```python
from build123d import *

# Parameters (mm, degrees)
SKETCH1_W           = 114.3
SKETCH1_H           = 35.814
BOSS_EXTRUDE1_DEPTH = 3.175
SKETCH3_R           = 1.8288
CUT_EXTRUDE2_DEPTH  = 4.175
SKETCH4_W           = 12.7
SKETCH4_H           = 35.814
CUT_EXTRUDE3_DEPTH  = 4.175
SKETCH5_R           = 1.8288
CUT_EXTRUDE4_DEPTH  = 4.175
BOSS_EXTRUDE4_DEPTH = 3.175
SKETCH9_R           = 1.8288
CUT_EXTRUDE5_DEPTH  = 4.175
BOSS_EXTRUDE5_DEPTH = 3.175


with BuildPart() as part:
    # Sketch1 → Boss-Extrude1 (new body)
    with BuildSketch(Plane(origin=(0, 0, 0), x_dir=(1, 0, 0), z_dir=(0, 1, 0))):
        Rectangle(SKETCH1_W, SKETCH1_H)
    extrude(amount=BOSS_EXTRUDE1_DEPTH)

    # Sketch3 → Cut-Extrude2 (cut, through all)
    with BuildSketch(Plane(origin=(0, 3.175, 0), x_dir=(1, 0, 0), z_dir=(0, 1, 0))):
        with Locations((-53.975, 14.986)):
            Circle(SKETCH3_R)
        with Locations((-53.975, -4.572)):
            Circle(SKETCH3_R)
        with Locations((-44.196, 12.319)):
            Circle(SKETCH3_R)
        with Locations((-44.196, -14.6304)):
            Circle(SKETCH3_R)
        with Locations((44.196, -14.6304)):
            Circle(SKETCH3_R)
        with Locations((53.975, -4.572)):
            Circle(SKETCH3_R)
        with Locations((44.196, 12.319)):
            Circle(SKETCH3_R)
        with Locations((53.975, 14.986)):
            Circle(SKETCH3_R)
    extrude(amount=-CUT_EXTRUDE2_DEPTH, mode=Mode.SUBTRACT)

    # Sketch4 → Cut-Extrude3 (cut, through all)
    with BuildSketch(Plane(origin=(0, 3.175, 0), x_dir=(1, 0, 0), z_dir=(0, 1, 0))):
        with Locations((50.8, 0)):
            Rectangle(SKETCH4_W, SKETCH4_H)
    extrude(amount=-CUT_EXTRUDE3_DEPTH, mode=Mode.SUBTRACT)

    # Sketch5 → Cut-Extrude4 (cut, through all)
    with BuildSketch(Plane(origin=(0, 3.175, 0), x_dir=(1, 0, 0), z_dir=(0, 1, 0))):
        with Locations((-44.196, 12.319)):
            Circle(SKETCH5_R)
        with Locations((-53.975, 14.986)):
            Circle(SKETCH5_R)
        with Locations((-53.975, -4.572)):
            Circle(SKETCH5_R)
        with Locations((-44.196, -14.6304)):
            Circle(SKETCH5_R)
        with Locations((31.496, -14.6304)):
            Circle(SKETCH5_R)
        with Locations((41.275, -4.572)):
            Circle(SKETCH5_R)
        with Locations((31.496, 12.319)):
            Circle(SKETCH5_R)
        with Locations((41.275, 14.986)):
            Circle(SKETCH5_R)
    extrude(amount=-CUT_EXTRUDE4_DEPTH, mode=Mode.SUBTRACT)

    # Sketch8 → Boss-Extrude4 (add)
    with BuildSketch(Plane(origin=(0, 3.175, 0), x_dir=(1, 0, 0), z_dir=(0, 1, 0))):
        with BuildLine():
            Line((44.196, 14.1478), (44.45, 14.542460619))
            Line((44.45, 14.542460619), (44.45, 10.507924783))
            ThreePointArc((44.45, 10.507924783), (42.371636577, 12.191691155), (44.196, 14.1478))
        make_face()
        with BuildLine():
            Line((44.196, -12.8016), (44.45, -12.55116419))
            Line((44.45, -12.55116419), (44.45, -16.7132))
            Line((44.45, -16.7132), (44.323, -16.5862))
            ThreePointArc((44.323, -16.5862), (42.3672, -14.7574), (44.196, -12.8016))
        make_face()
    extrude(amount=-BOSS_EXTRUDE4_DEPTH)

    # Sketch9 → Cut-Extrude5 (cut, through all)
    with BuildSketch(Plane(origin=(0, 3.175, 0), x_dir=(1, 0, 0), z_dir=(0, 1, 0))):
        with Locations((37.973, -4.572)):
            Circle(SKETCH9_R)
        with Locations((37.973, 14.986)):
            Circle(SKETCH9_R)
    extrude(amount=-CUT_EXTRUDE5_DEPTH, mode=Mode.SUBTRACT)

    # Sketch10 → Boss-Extrude5 (add)
    with BuildSketch(Plane(origin=(0, 3.175, 0), x_dir=(1, 0, 0), z_dir=(0, 1, 0))):
        with BuildLine():
            ThreePointArc((39.624, 14.199419782), (39.8018, 14.986), (39.624, 15.772580218))
            ThreePointArc((39.624, 15.772580218), (43.1038, 14.986), (39.624, 14.199419782))
        make_face()
        with BuildLine():
            ThreePointArc((39.624, -5.358580218), (39.8018, -4.572), (39.624, -3.785419782))
            ThreePointArc((39.624, -3.785419782), (43.1038, -4.572), (39.624, -5.358580218))
        make_face()
    extrude(amount=-BOSS_EXTRUDE5_DEPTH)


solid = part.part
```
Build history of the part. All positions in model axes, mm. Give positions to 0.01 mm unless a question says otherwise; leave off trailing zeros. Return JSON: item names as keys, results as strings.
Q1. Flat gauge pin, fed straight in: pin 1 (3 mm diameter, centred on x = -53.975, z = -14.986, fed in from -Y). Where does the tip first touch, or does it go through?
Answer list:
{"pin 1": "passes through"}
Q2. Two-plate mould, pull along X, no slides. Class faces 1 (the face through (-6, 0, 0)), 2 (the face through (-57.15, 2, 0)), 3 (the face through (30.148, 1.61, -13.555)): pulls with the +X half, pulls with the -X half, needs draft (parallel to the pull), parting line crosses it, or undercut.
Answer list:
{"face 1": "needs draft", "face 2": "pulls with the -X half", "face 3": "undercut"}
Q3. Band-saw the part on A-A (y = 1.2). Count the separate pieces of the cut face and the enclosed holes in it, then the cut area to 3 significant figures.
Answer list:
{"separate pieces": "1", "enclosed holes": "9", "area": "3,550 mm^2"}
Q4. Wall check: probe 1 along Z at (x, y) = (38, 1.1); probe 2 along X at (y, z) = (0.65, -12.5); probe 3 along X at (y, z) = (0.8, 5). Give the ranges that are in metal, low to high. Write a range as from..to.
Answer list:
{"probe 1": "z = -17.91..-16.81, -13.16..2.74, 6.4..17.91", "probe 2": "x = -57.15..-46.02, -42.38..29.68, 33.32..44.45", "probe 3": "x = -57.15..-55.75, -52.2..36.19, 39.75..44.45"}
